Work out the finished part from the listing and answer in its coordinate system (mm). A direction names the side the tool comes from. Coordinates: 2 decimals unless noted, no trailing zeros. Write each loop counter-clockwise with the first axis right and the second up, starting at its lowest first coordinate (ties: lowest second). Pieces come first, ordered by that corner, then holes. Notation, with made-up numbers: (-10, -7.75) - (41, -7.75) arc R20 ccw to (41, 3.25) - close; hole circle Ø7 at (-27.75, -36). An arc over 180 degrees is marked (long way). Use a Markdown table: item, result. Add a question column.
(1) For a pull along Y with two mould halves and no side action, classify faces 1 (the face through (-14.8, 2.49, 28.17)), 2 (the face through (16.979, 2.967, -11.458)), 3 (the face through (11, 3, 26)), 4 (the face through (16, 5.5, -15)) as released by +Y, released by -Y, zero draft, split by the parting line, or undercut.
(2) The part is cut by section B-B, the plane z = 9.5. Give the vertices of the cut face in (x, y).
(3) Find the intervals of material crossed by line 1 (X direction, y = 0.5, z = 29); line 2 (Z direction, x = 1.5, y = 3.5); line 3 (Y direction, x = -13, z = -7), in increasing order. Write a range as from..to.
(4) Given pin 1 Ø1.5 at (x, y) = (13, 1) entering from -Z; pin 2 Ø1.8 at (x, z) = (16.5, -14) entering from -Y; pin 3 Ø2 at (x, y) = (6, 5.5) entering from +Z, each flat-ended and moving along its own axis, determine where each tip first touches the part or whether it passes through.
(5) A tool of negligible diameter and unlimited length cuts with its end or side. For faces 5 (the face through (11.5, 3, -32)), 6 (the face through (0, 3, -24.207)), 7 (the face through (-11.5, 3, -32)), from which of +Z, -Z, +X, -X, +Y, -Y can it reach the whole face along a straight path? Write none if from no direction.
(6) The part is cut by section A-A, the plane z = -25.5. Give the vertices of the cut face in (x, y), then the cut area to 3 significant figures.
Autodesk Inventor part; units mm, degrees
ref_plane "YZ Plane" through (0, 0, 0) normal (1, 0, 0) x (0, 1, 0)
ref_plane "XZ Plane" through (0, 0, 0) normal (0, 1, 0) x (-1, 0, 0)
ref_plane "XY Plane" through (0, 0, 0) normal (0, 0, 1) x (1, 0, 0)
sketch "Sketch1" plane through (0, 0, 0) normal (0, 1, 0) x (-1, 0, 0)
  line L0 (11, 32.7929) -> (11, 17.7929)
  line L1 (11, 17.7929) -> (-2.062, 17.7929)
  line L2 (11, 32.7929) -> (18.5, 32.7929)
  line L3 (18.5, 32.7929) -> (18.5, 17.7929)
  line L4 (18.5, 17.7929) -> (11.5, -24.2071)
  line L5 (11.5, -24.2071) -> (11.5, -39.2071)
  line L6 (11.5, -39.2071) -> (5.7, -39.2071)
  line L7 (5.7, -39.2071) -> (5.7, -24.2071)
  line L8 (5.7, -24.2071) -> (0.6352, -24.2071)
  line L9 (0, 0) -> (0, 4.5611)
  line L10 (-11, 32.7929) -> (-11, 17.7929)
  line L11 (-11, 17.7929) -> (-2.062, 17.7929)
  line L12 (-11, 32.7929) -> (-18.5, 32.7929)
  line L13 (-18.5, 32.7929) -> (-18.5, 17.7929)
  line L14 (-18.5, 17.7929) -> (-11.5, -24.2071)
  line L15 (-11.5, -24.2071) -> (-11.5, -39.2071)
  line L16 (-11.5, -39.2071) -> (-5.7, -39.2071)
  line L17 (-5.7, -39.2071) -> (-5.7, -24.2071)
  line L18 (-5.7, -24.2071) -> (0.6352, -24.2071)
  dimension "d0" = 37
  dimension "d1" = 7.5
  dimension "d2" = 15
  dimension "d3" = 5.8
  dimension "d4" = 23
  dimension "d5" = 72
  dimension "d6" = 15
  dimension "d7" = 15
  dimension "d8" = 15
extrude "Extrusion1" add sketch "Sketch1" along normal blind 6
sketch "Sketch2" plane through (0, 6, 0) normal (0, 1, 0) x (1, 0, 0)
  line L0 (-11, -17.7929) -> (11, -17.7929)
  line L1 (18.5, -17.7929) -> (11.5, 24.2071)
  line L2 (5.7, 24.2071) -> (-5.7, 24.2071)
  line L3 (-11.5, 24.2071) -> (-18.5, -17.7929)
  line L4 (-14.9586, -14.7929) -> (-8.9586, 21.2071)
  line L5 (-8.9586, 21.2071) -> (8.9586, 21.2071)
  line L6 (8.9586, 21.2071) -> (14.9586, -14.7929)
  line L7 (14.9586, -14.7929) -> (-14.9586, -14.7929)
  point P0 (0, 0)
  dimension "d11" = 3
  dimension "d12" = 3
  dimension "d13" = 3
  dimension "d14" = 3
extrude "Extrusion2" cut sketch "Sketch2" against normal blind 6
sketch "Sketch3" plane through (-5.7, 0, -24.2071) normal (1, 0, 0) x (0, 0, -1)
  line L0 (15, 0) -> (15, 6)
  circle A0 centre (12, 3) radius 1.7
  point P0 (-24.2071, 0)
  dimension "d17" = 3.4
  dimension "d18" = 3
extrude "Extrusion3" cut sketch "Sketch3" along normal through all both and the other way through all
sketch "Sketch4" plane through (18.5, 0, 32.7929) normal (1, 0, 0) x (0, 0, -1)
  line L0 (0, 0) -> (0, 6)
  circle A0 centre (3, 3) radius 3.75
  point P0 (32.7929, 0)
  dimension "d21" = 7.5
  dimension "d22" = 3
extrude "Extrusion4" add sketch "Sketch4" against normal up to surface (7.5 mm away)
sketch "Sketch5" plane through (18.5, 0, 17.7929) normal (1, 0, 0) x (0, 0, -1)
  line L0 (-15, 6) -> (-14.25, 6)
  line L1 (-15, 0) -> (-15, 0.75)
  line L2 (-15, 0) -> (-14.25, 0)
  line L3 (-15, 5.25) -> (-15, 6)
  line L4 (-15, 6) -> (-14.25, 6)
  line L5 (-15, 0.75) -> (-15, 0)
  line L6 (-15, 0) -> (-14.25, 0)
  arc A0 (-14.25, 6) -> (-15, 5.25) centre (-12, 3) ccw
  arc A1 (-15, 0.75) -> (-14.25, 0) centre (-12, 3) ccw
  point P0 (17.7929, 0)
extrude "Extrusion5" cut sketch "Sketch5" against normal through all
sketch "Sketch6" plane through (-11, 0, 17.7929) normal (1, 0, 0) x (0, 0, -1)
  arc A0 (-15, 0.75) -> (-14.25, 0) centre (-12, 3) ccw
  circle A1 centre (-12, 3) radius 3.75
  point P0 (17.7929, 0)
  dimension "d27" = 7.5
extrude "Extrusion6" add sketch "Sketch6" against normal up to surface (7.5 mm away)
hole "Hole1" at (18.5, 3, 29.7929) direction (-1, 0, 0) diameter 3.4 depth 46.75 tip angle 118
ref_plane "Work Plane1" through (18.5, 0, -39.2071) normal (-1, 0, 0) x (0, 0, 1)
sketch "Sketch7" plane through (18.5, 0, -39.2071) normal (-1, 0, 0) x (0, 0, 1)
  line L0 (27, 3) -> (21, 3) construction
  line L1 (27, 0.5) -> (21, 0.5)
  line L2 (21, 5.5) -> (27, 5.5)
  arc A0 (27, 0.5) -> (27, 5.5) centre (27, 3) ccw
  arc A1 (21, 5.5) -> (21, 0.5) centre (21, 3) ccw
  circle A2 centre (3, 3) radius 1.7
  line L3 (15, 0) -> (15, 6)
  point P0 (39.2071, 0)
  point P1 (24, 3)
  point P2 (15, 3)
  dimension "d40" = 21
  dimension "d41" = 5
  dimension "d42" = 6
extrude "Extrusion7" add sketch "Sketch7" along normal blind 7.25 contours L1 A1 L2 A0
sketch "Sketch8" plane through (18.5, 0, -39.2071) normal (1, 0, 0) x (0, 0, -1)
  arc A0 (-21, 0.5) -> (-21, 5.5) centre (-21, 3) ccw
  arc A1 (-27, 5.5) -> (-27, 0.5) centre (-27, 3) ccw
  point P0 (-39.2071, 0)
hole "Hole2" at (18.5, 3, -12.2071) at (18.5, 3, -18.2071) direction (-1, 0, 0) diameter 1.5 depth 3 tip angle 118
sketch "Sketch9" plane through (18.5, 0, -39.2071) normal (1, 0, 0) x (0, 0, -1)
  arc A0 (-21, 0.5) -> (-21, 5.5) centre (-21, 3) ccw
  arc A1 (-27, 5.5) -> (-27, 0.5) centre (-27, 3) ccw
  line L0 (-27, 3) -> (-21, 3)
  point P0 (-39.2071, 0)
  point P1 (-24, 3)
hole "Hole3" at (18.5, 3, -15.2071) direction (-1, 0, 0) diameter 2.459 depth 10.8 tip angle 118
equation "\"d8\" = d7"
properties part number "500-006" material "ABS Plastic"
Model answer:
| question | item | result |
|---|---|---|
| 1 | face 1 | undercut |
| 1 | face 2 | undercut |
| 1 | face 3 | zero draft |
| 1 | face 4 | released by +Y |
| 2 | outline | (-17.12, 0) - (-14.08, 0) - (-14.08, 6) - (-17.12, 6) - close; (14.08, 0) - (17.12, 0) - (17.12, 6) - (14.08, 6) - close |
| 3 | line 1 | -18.5..-11, 11..18.5 |
| 3 | line 2 | -24.21..-21.21, 14.79..17.79 |
| 3 | line 3 | 0..6 |
| 4 | pin 1 | z = -20.37 |
| 4 | pin 2 | y = 0.5 |
| 4 | pin 3 | z = 17.79 |
| 5 | face 5 | -Z, +X, +Y, -Y |
| 5 | face 6 | -Z, +Y, -Y |
| 5 | face 7 | -Z, -X, +Y, -Y |
| 6 | outline | (-11.5, 0) - (-5.7, 0) - (-5.7, 6) - (-11.5, 6) - close; (5.7, 0) - (11.5, 0) - (11.5, 6) - (5.7, 6) - close |
| 6 | area | 69.6 mm^2 |
